from build123d import *

# Parameters (mm, degrees)
F0_R     = 260
F1_DEPTH = 25.4
F2_R     = 12.69999
F3_R     = 4
F4_DEPTH = 19.05
F5_DEPTH = 19.05


# Not quite as in the source:
# - a fillet or chamfer is up to 0.001 mm smaller than in the source, because OpenCascade refuses the exact size


with BuildPart() as f1:
    # F0 (on Top) → F1 (new body)
    with BuildSketch(Plane.XY):
        Circle(F0_R)
    extrude(amount=F1_DEPTH)

    # F2 (radius 12.7 in the source; OpenCascade refuses exactly that, so slightly less here)
    f2_edges = [f1.edges().sort_by_distance(p)[0] for p in [
        (-260, 0, 25.4),
        (-260, 0, 0),
    ]]
    fillet(f2_edges, radius=F2_R)

    # F3 (on face) → F4 (cut)
    with BuildSketch(Plane(origin=(0, 0, 0), x_dir=(1, 0, 0), z_dir=(0, 0, -1))):
        with Locations((160.0338797814, 166.028664158)):
            Circle(F3_R)
    extrude(amount=-F4_DEPTH, mode=Mode.SUBTRACT)

    # F3 (on face) → F5 (cut)
    with BuildSketch(Plane(origin=(0, 0, 0), x_dir=(1, 0, 0), z_dir=(0, 0, -1))):
        with Locations((-160.0338797814, 166.028664158)):
            Circle(F3_R)
        with Locations((160.0338797814, 166.028664158)):
            Circle(F3_R)
        with Locations((160.0338797814, -166.028664158)):
            Circle(F3_R)
        with Locations((-160.0338797814, -166.028664158)):
            Circle(F3_R)
    extrude(amount=-F5_DEPTH, mode=Mode.SUBTRACT)


solid = f1.part
Can you work these out from the model? Positions are in its coordinate system, mm. Give positions to 0.01 mm unless a question says otherwise; leave off trailing zeros. Order: outer loops, then holes, each group sorted by start corner. A loop starts at its lowest first (then second) coordinate and runs counter-clockwise, first axis right, second up. Notation, with made-up numbers: M 85,-9 L 132,-9 A14 cw 132,12 Z; hole C -11,44 d4. An arc over 180 degrees is marked long. One line per item, written item: value.
Item 1: Please list where these lines run through material, in increasing order: line 1 (Y direction, x = 2, z = 14); line 2 (X direction, y = 178, z = 10.75); line 3 (X direction, y = -70, z = 23.25).
Verdict:
line 1: -259.93 to 259.93
line 2: -189.31 to 189.31
line 3: -244.55 to 244.55
Item 2: If we section it at A-A on z = 6.75: Write out the boundary of the cut face in (x, y).
Verdict:
outline: C 0,0 d517.04; hole C -160.03,-166.03 d8; hole C -160.03,166.03 d8; hole C 160.03,-166.03 d8; hole C 160.03,166.03 d8
Item 3: For pin 1 (6.5 mm diameter, centred on x = 161, y = 167, fed in from -Z); pin 2 (2 mm diameter, centred on x = 193.5, z = 4.5, fed in from -Y); pin 3 (6 mm diameter, centred on x = -71, z = 21, fed in from -Y); pin 4 (5 mm diameter, centred on x = 160.03, y = -166.03, fed in from -Z), each with a flat end and sliding along its axis, tell me the tip position at first contact or that it passes through.
Verdict:
pin 1: z = 0
pin 2: y = -170.78
pin 3: y = -249.14
pin 4: z = 19.05
